The listing builds one solid part. Answer for the finished solid, in the listing's coordinates (mm). Give positions to 0.01 mm unless a question says otherwise; leave off trailing zeros. Order: outer loops, then holes, each group sorted by start corner. A loop starts at its lowest first (then second) coordinate and runs counter-clockwise, first axis right, second up. Notation, with made-up numbers: (20.5, 87.25) - (50.5, 87.25) arc R25 cw to (50.5, 117.25) - close; hole circle Ø3 at (-11.5, 52.5). An arc over 180 degrees is marked (long way). Answer in a Markdown table with one row per item. Add a question column.
```python
from build123d import *

# Parameters (mm, degrees)
SKETCH_1_R          = 2.2
EXTRUDE_1_DEPTH     = 5
SKETCH_2_W          = 5
SKETCH_2_H          = 220.282443136
SKETCH_2_H_2        = 219.868690955
CUT_EXTRUDE_1_DEPTH = 10
SKETCH_3_W          = 5
SKETCH_3_H          = 40
EXTRUDE_3_DEPTH     = 5
SKETCH_4_W          = 390.4211829
SKETCH_4_H          = 264.690207343
EXTRUDE_4_DEPTH     = 5
SKETCH_5_R          = 2.2
CUT_EXTRUDE_2_DEPTH = 5
SKETCH_6_W          = 410
SKETCH_6_H          = 266.694039068
CUT_EXTRUDE_4_DEPTH = 10


with BuildPart() as part:
    # 草图1 → 凸台-拉伸1 (new body)
    with BuildSketch(Plane.XY):
        Polygon((-200, 150), (200, 150), (200, 110), (205, 110), (205, 70), (200, 70), (200, 30), (205, 30), (205, -30), (200, -30), (200, -70), (205, -70), (205, -110), (200, -110), (200, -150), (160, -150), (160, -155), (120, -155), (120, -150), (80, -150), (80, -155), (40, -155), (40, -150), (-40, -150), (-40, -155), (-80, -155), (-80, -150), (-120, -150), (-120, -155), (-160, -155), (-160, -150), (-200, -150), (-200, -110), (-205, -110), (-205, -70), (-200, -70), (-200, -30), (-205, -30), (-205, 30), (-200, 30), (-200, 70), (-205, 70), (-205, 110), (-200, 110), align=None)
        with Locations((-140, -140)):
            Circle(SKETCH_1_R, mode=Mode.SUBTRACT)
        with Locations((-100, -140)):
            Circle(SKETCH_1_R, mode=Mode.SUBTRACT)
        with Locations((-60, -140)):
            Circle(SKETCH_1_R, mode=Mode.SUBTRACT)
        with Locations((-20, -140)):
            Circle(SKETCH_1_R, mode=Mode.SUBTRACT)
        with Locations((20, -140)):
            Circle(SKETCH_1_R, mode=Mode.SUBTRACT)
        with Locations((60, -140)):
            Circle(SKETCH_1_R, mode=Mode.SUBTRACT)
        with Locations((100, -140)):
            Circle(SKETCH_1_R, mode=Mode.SUBTRACT)
        with Locations((140, -140)):
            Circle(SKETCH_1_R, mode=Mode.SUBTRACT)
        with Locations((-190, 110)):
            Circle(SKETCH_1_R, mode=Mode.SUBTRACT)
        with Locations((-190, 70)):
            Circle(SKETCH_1_R, mode=Mode.SUBTRACT)
        with Locations((-190, 30)):
            Circle(SKETCH_1_R, mode=Mode.SUBTRACT)
        with Locations((-190, -30)):
            Circle(SKETCH_1_R, mode=Mode.SUBTRACT)
        with Locations((-190, -70)):
            Circle(SKETCH_1_R, mode=Mode.SUBTRACT)
        with Locations((-190, -110)):
            Circle(SKETCH_1_R, mode=Mode.SUBTRACT)
        with Locations((190, -110)):
            Circle(SKETCH_1_R, mode=Mode.SUBTRACT)
        with Locations((190, -70)):
            Circle(SKETCH_1_R, mode=Mode.SUBTRACT)
        with Locations((190, -30)):
            Circle(SKETCH_1_R, mode=Mode.SUBTRACT)
        with Locations((190, 30)):
            Circle(SKETCH_1_R, mode=Mode.SUBTRACT)
        with Locations((190, 70)):
            Circle(SKETCH_1_R, mode=Mode.SUBTRACT)
        with Locations((190, 110)):
            Circle(SKETCH_1_R, mode=Mode.SUBTRACT)
    extrude(amount=EXTRUDE_1_DEPTH)

    # 草图2 → 切除-拉伸1 (cut)
    with BuildSketch(Plane.XY.offset(5)):
        with Locations((-202.5, -0.141221568)):
            Rectangle(SKETCH_2_W, SKETCH_2_H)
        with Locations((202.5, 0.065654522)):
            Rectangle(SKETCH_2_W, SKETCH_2_H_2)
    extrude(amount=-CUT_EXTRUDE_1_DEPTH, mode=Mode.SUBTRACT)

    # 草图3 → 凸台-拉伸3 (add)
    with BuildSketch(Plane.XY.offset(5)):
        with Locations((-202.5, 130)):
            Rectangle(SKETCH_3_W, SKETCH_3_H)
        with Locations((-202.5, 50)):
            Rectangle(SKETCH_3_W, SKETCH_3_H)
        with Locations((-202.5, -50)):
            Rectangle(SKETCH_3_W, SKETCH_3_H)
        with Locations((-202.5, -130)):
            Rectangle(SKETCH_3_W, SKETCH_3_H)
        with Locations((202.5, -130)):
            Rectangle(SKETCH_3_W, SKETCH_3_H)
        with Locations((202.5, -50)):
            Rectangle(SKETCH_3_W, SKETCH_3_H)
        with Locations((202.5, 50)):
            Rectangle(SKETCH_3_W, SKETCH_3_H)
        with Locations((202.5, 130)):
            Rectangle(SKETCH_3_W, SKETCH_3_H)
    extrude(amount=-EXTRUDE_3_DEPTH)

    # 草图4 → 凸台-拉伸4 (add)
    with BuildSketch(Plane.XY.offset(5)):
        with Locations((1.806920954, 7.46039962)):
            Rectangle(SKETCH_4_W, SKETCH_4_H)
    extrude(amount=-EXTRUDE_4_DEPTH)

    # 草图5 → 切除-拉伸2 (cut)
    with BuildSketch(Plane.XY.offset(5)):
        with Locations((-190, 90)):
            Circle(SKETCH_5_R)
        with Locations((-190, 50)):
            Circle(SKETCH_5_R)
        with Locations((-190, 0)):
            Circle(SKETCH_5_R)
        with Locations((-190, -50)):
            Circle(SKETCH_5_R)
        with Locations((-190, -90)):
            Circle(SKETCH_5_R)
        with Locations(Location((190, -90, 0), (0, 0, 180))):
            Circle(SKETCH_5_R)
        with Locations(Location((190, -50, 0), (0, 0, 180))):
            Circle(SKETCH_5_R)
        with Locations(Location((190, 0, 0), (0, 0, 180))):
            Circle(SKETCH_5_R)
        with Locations(Location((190, 50, 0), (0, 0, 180))):
            Circle(SKETCH_5_R)
        with Locations(Location((190, 90, 0), (0, 0, 180))):
            Circle(SKETCH_5_R)
    extrude(amount=-CUT_EXTRUDE_2_DEPTH, mode=Mode.SUBTRACT)

    # 草图6 → 切除-拉伸4 (cut)
    with BuildSketch(Plane.XY.offset(5)):
        with Locations((0, 63.347019534)):
            Rectangle(SKETCH_6_W, SKETCH_6_H)
    extrude(amount=-CUT_EXTRUDE_4_DEPTH, mode=Mode.SUBTRACT)


solid = part.part
```
(1) Each of these flat-tipped pins is pushed along its axis until it touches: P1, Ø3, axis at y = -78.5, z = 2.5, coming from the -X side; P2, Ø2.5, axis at x = -203, z = 2.5, coming from the +Y side; P3, Ø3.5, axis at x = -190, y = -90, coming from the -Z side; P4, Ø1.5, axis at y = -152.5, z = 1.5, coming from the +X side. Where does it stop, or does it pass through?
(2) Find section C-C, the plane y = -74.5. Write down the section's boundary in (x, z).
(3) Find section A-A, the plane z = 2.2. Give the number of separate pieces and of enclosed holes in the cut face, plus the area to 3 significant figures.
(4) Find section B-B, the plane x = 33.5. Write down the section's boundary in (y, z).
(5) Straight lines are drawn through the part: line 1 (Y direction, x = 100, z = 1.5); line 2 (Y direction, x = 190, z = 2.35); line 3 (X direction, y = -91.5, z = 0.9). For each, find the intervals that lie inside material, in ascending order.
Answer key:
| question | item | result |
|---|---|---|
| 1 | P1 | x = -200 |
| 1 | P2 | y = -110 |
| 1 | P3 | through |
| 1 | P4 | x = 160 |
| 2 | outline | (-200, 0) - (200, 0) - (200, 5) - (-200, 5) - close |
| 3 | separate pieces | 1 |
| 3 | enclosed holes | 10 |
| 3 | area | 33,000 mm² |
| 4 | outline | (-150, 0) - (-70, 0) - (-70, 5) - (-150, 5) - close |
| 5 | line 1 | -150 to -142.2, -137.8 to -70 |
| 5 | line 2 | -150 to -92.2, -87.8 to -70 |
| 5 | line 3 | -200 to -191.61, -188.39 to 188.39, 191.61 to 200 |
